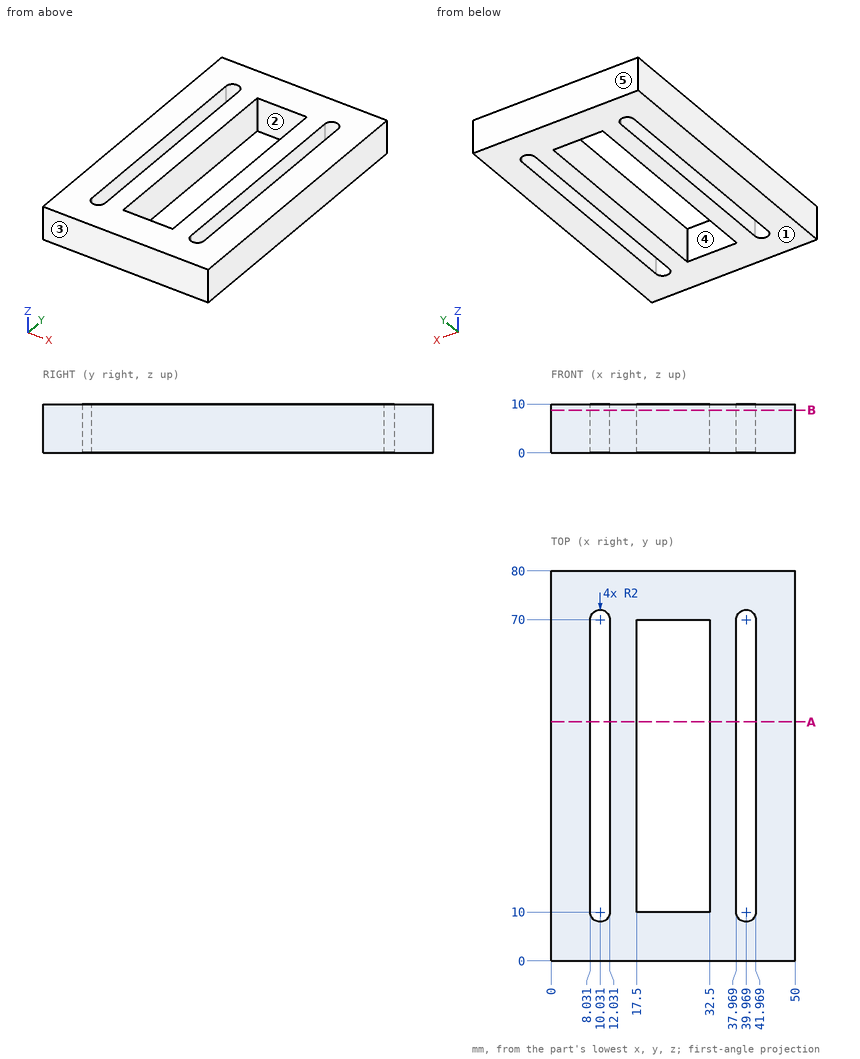
Here's the drawing with two shaded views (mm, measured from the low corner). I have some questions. A direction names the side the tool comes from. Coordinates: 2 decimals unless noted, no trailing zeros. Write each loop counter-clockwise with the first axis right and the second up, starting at its lowest first coordinate (ties: lowest second). Pieces come first, ordered by that corner, then holes.
Item 1: Will these pins go through, and if not, where does the flat tip stop? pin 1 (4 mm diameter, centred on x = 9, z = 1, fed in from -Y); pin 2 (1 mm diameter, centred on x = 19, y = 52, fed in from +Z).
Item 2: If I drill on line 1 (X direction, y = 65, z = 9); line 2 (Y direction, x = 20, z = 9.25); line 3 (Y direction, x = 41.5, z = 9), over which ranges is the centre line in solid material (lowest first)?
Item 3: I want a section at B-B on z = 8.75. Write out the boundary of the cut face in (x, y), and give its area (4 significant figures).
Item 4: On a 3-axis mill with a long thin cutter (end or side, diameter ignored), from which of +Z, -Z, +X, -X, +Y, -Y can I reach the whole of each face in a straight line? I mean the marked faces 4 and 5. Say none if no direction works.
Item 5: I want a section at A-A on y = 49. Write out the boundary of the cut face in (x, z), and give its area (3 significant figures).
Item 6: If we mould it in two halves opening along Y, with no side actions, what happens to the marked faces 1, 2 and 3? For each: +Y half, -Y half, draft (parallel to the pull), parting line (faces both ways), or undercut.
Findings below:
1. pin 1: stops at y = 0
1. pin 2: passes through
2. line 1: x = 0 to 8.03, 12.03 to 17.5, 32.5 to 37.97, 41.97 to 50
2. line 2: y = 0 to 10, 70 to 80
2. line 3: y = 0 to 8.71, 71.29 to 80
3. outline: (0, 0) - (50, 0) - (50, 80) - (0, 80) - close; hole (8.03, 10) arc R2 ccw to (12.03, 10) - (12.03, 70) arc R2 ccw to (8.03, 70) - close; hole (17.5, 10) - (32.5, 10) - (32.5, 70) - (17.5, 70) - close; hole (37.97, 10) arc R2 ccw to (41.97, 10) - (41.97, 70) arc R2 ccw to (37.97, 70) - close
3. area: 2,595 mm2
4. face 4: +Z, -Z
4. face 5: +Z, -Z, +X, -X, +Y
5. outline: (0, 0) - (8.03, 0) - (8.03, 10) - (0, 10) - close; (12.03, 0) - (17.5, 0) - (17.5, 10) - (12.03, 10) - close; (32.5, 0) - (37.97, 0) - (37.97, 10) - (32.5, 10) - close; (41.97, 0) - (50, 0) - (50, 10) - (41.97, 10) - close
5. area: 270 mm2
6. face 1: draft
6. face 2: undercut
6. face 3: -Y half
